```python
from build123d import *

# Parameters (mm, degrees)
SKETCH1_W               = 45.72
SKETCH1_H               = 17.78
BOSS_EXTRUDE1_DEPTH     = 45.72
SKETCH2_W               = 38.1
SKETCH2_H               = 12.7
CUT_EXTRUDE1_DEPTH      = 41.91
SKETCH6_R               = 3.048
CUT_EXTRUDE2_DEPTH      = 1.512975339
CUT_EXTRUDE2_DEPTH_BACK = 15.24


with BuildPart() as part:
    # Sketch1 → Boss-Extrude1 (new body)
    with BuildSketch(Plane(origin=(0, 0, 0), x_dir=(1, 0, 0), z_dir=(0, 1, 0))):
        with Locations((22.86, 8.89)):
            Rectangle(SKETCH1_W, SKETCH1_H)
    extrude(amount=BOSS_EXTRUDE1_DEPTH)

    # Sketch2 → Cut-Extrude1 (cut)
    with BuildSketch(Plane(origin=(0, 45.72, 0), x_dir=(1, 0, 0), z_dir=(0, 1, 0))):
        with Locations((22.86, 8.89)):
            Rectangle(SKETCH2_W, SKETCH2_H)
    extrude(amount=-CUT_EXTRUDE1_DEPTH, mode=Mode.SUBTRACT)

    # Sketch6 → Cut-Extrude2 (cut, two sides)
    with BuildSketch(Plane(origin=(0, 0, 0), x_dir=(-0.983268965, 0.18208123, 0.005344962), z_dir=(-0.182159664, -0.982845594, -0.028851256))) as cut_extrude2_sk:
        with Locations((-22.14222649, 8.882344385)):
            Circle(SKETCH6_R)
        with Locations((-15.03022649, 8.882344385)):
            Circle(SKETCH6_R)
        with Locations((-29.25422649, 8.882344385)):
            Circle(SKETCH6_R)
    extrude(amount=CUT_EXTRUDE2_DEPTH, mode=Mode.SUBTRACT)
    extrude(cut_extrude2_sk.sketch, amount=-CUT_EXTRUDE2_DEPTH_BACK, mode=Mode.SUBTRACT)


solid = part.part
```
Build history of the part. All positions in model axes, mm. A direction names the side the tool comes from. Round coordinates to 2 decimals unless told otherwise and drop trailing zeros. Loops run counter-clockwise (first coordinate to the right, second up) from the corner with the lowest first, then second, coordinate; pieces in that order, holes last. Notation, with made-up numbers: M 29,-26 L 34,-26 A32 cw 34,8 Z; hole C 2,48.5 d7. An arc over 180 degrees is marked long. Answer as CSV lines item,"result".
1. Cut at C-C on z = -12.5. Write the cut outline in (x, y).
Resolved:
outline,"M 0,0 L 45.72,0 L 45.72,45.72 L 41.91,45.72 L 41.91,3.81 L 3.81,3.81 L 3.81,45.72 L 0,45.72 Z"
2. Wall check: probe 1 along X at (y, z) = (23, -9.5); probe 2 along Z at (x, y) = (26, 38.5); probe 3 along Y at (x, z) = (21, -12.25). Give the ranges that are in metal, low to high. Write a range as [from, to].
Resolved:
probe 1,"x = [0, 3.81], [41.91, 45.72]"
probe 2,"z = [-17.78, -15.24], [-2.54, 0]"
probe 3,"y = [0, 3.81]"
3. Cut at D-D on z = -10. Count the separate pieces of the cut face and the enclosed holes in it, then the cut area to 3 significant figures.
Resolved:
separate pieces,"4"
enclosed holes,"0"
area,"428 mm²"
4. Cut at B-B on x = 36. Write the cut outline in (y, z).
Resolved:
outline,"M 0,-17.78 L 45.72,-17.78 L 45.72,-15.24 L 3.81,-15.24 L 3.81,-2.54 L 45.72,-2.54 L 45.72,0 L 0,0 Z"
5. 3-axis set-ups, long thin cutter, end or side, ignore diameter. For faces 4 (the flat face through (23, 0, -5)), 5 (the flat face through (23, 25, -15.24)): which of +Z, -Z, +X, -X, +Y, -Y reach the whole face in a straight line?
Resolved:
face 4,"+Z, -Z, +X, -X, -Y"
face 5,"+Y"
6. Flat gauge pin, fed straight in: P1, Ø4, axis at x = 25.5, z = -11.5, coming from the +Y side. Where does the tip first touch, or does it go through?
Resolved:
P1,"stops at y = 3.81"
7. Cut at A-A on y = 30.5. Write the cut outline in (x, z), then the cut area to 3 significant figures.
Resolved:
outline,"M 0,-17.78 L 45.72,-17.78 L 45.72,0 L 0,0 Z; hole M 3.81,-15.24 L 41.91,-15.24 L 41.91,-2.54 L 3.81,-2.54 Z"
area,"329 mm²"
8. Two-plate mould, pull along X, no slides. Class faces 1 (the flat face through (45.72, 23, -9)), 2 (the flat face through (23, 45.72, -17)), 3 (the flat face through (3.81, 25, -9)): released by +X, released by -X, zero draft, split by the parting line, or undercut.
Resolved:
face 1,"released by +X"
face 2,"zero draft"
face 3,"undercut"
